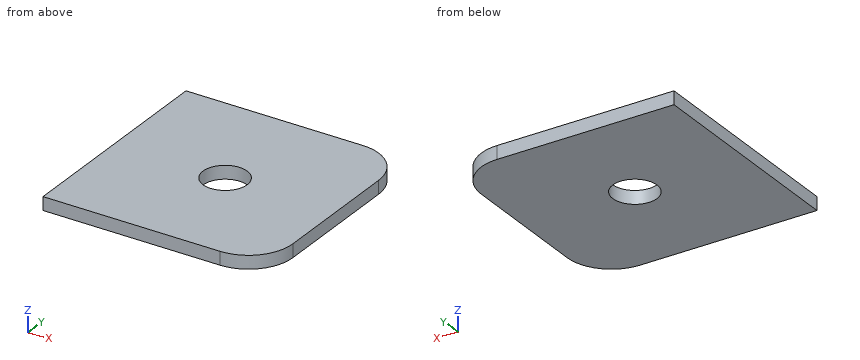
from build123d import *

# Parameters (mm, degrees)
SKETCH1_R           = 5
BOSS_EXTRUDE1_DEPTH = 3


with BuildPart() as part:
    # Sketch1 → Boss-Extrude1 (new body)
    with BuildSketch(Plane.XY):
        with BuildLine():
            Line((-24.011627907, 26.308139535), (15.988372093, 26.308139535))
            ThreePointArc((15.988372093, 26.308139535), (23.059439905, 23.379207347), (25.988372093, 16.308139535))
            Line((25.988372093, 16.308139535), (25.988372093, -13.691860465))
            ThreePointArc((25.988372093, -13.691860465), (23.059439905, -20.762928277), (15.988372093, -23.691860465))
            Line((15.988372093, -23.691860465), (-24.011627907, -23.691860465))
            Line((-24.011627907, -23.691860465), (-24.011627907, 26.308139535))
        make_face()
        with Locations((0.988372093, 1.308139535)):
            Circle(SKETCH1_R, mode=Mode.SUBTRACT)
    extrude(amount=BOSS_EXTRUDE1_DEPTH)


solid = part.part
The listing builds one solid part. Answer for the finished solid, in the listing's coordinates (mm). Round coordinates to 2 decimals unless told otherwise and drop trailing zeros. Order: outer loops, then holes, each group sorted by start corner. A loop starts at its lowest first (then second) coordinate and runs counter-clockwise, first axis right, second up. Notation, with made-up numbers: (37.5, 51.25) -> (94.5, 51.25) arc R7 cw to (94.5, 60.25) -> close; hole circle Ø10 at (-33, -19). An arc over 180 degrees is marked (long way). One line per item, written item: value.
Item 1: Straight lines are drawn through the part: L1, parallel to Y at x = 1, z = 0.9; L2, parallel to Y at x = 3, z = 0.2; L3, parallel to X at y = 19, z = 0.65. For each, find the intervals that lie inside material, in ascending order.
Taken from the geometry:
L1: y = -23.69 to -3.69, 6.31 to 26.31
L2: y = -23.69 to -3.27, 5.89 to 26.31
L3: x = -24.01 to 25.62
Item 2: Find section A-A, the plane z = 0.8. Give the vertices of the cut face in (x, y).
Taken from the geometry:
outline: (-24.01, -23.69) -> (15.99, -23.69) arc R10 ccw to (25.99, -13.69) -> (25.99, 16.31) arc R10 ccw to (15.99, 26.31) -> (-24.01, 26.31) -> close; hole circle Ø10 at (0.99, 1.31)
Item 3: Find section B-B, the plane x = 19.5. Give the vertices of the cut face in (y, z) (3 decimals), then the cut area to 3 significant figures.
Taken from the geometry:
outline: (-23.055, 0) -> (25.671, 0) -> (25.671, 3) -> (-23.055, 3) -> close
area: 146 mm2
